Design review of the part built by this model. Coordinates are the model's own, in mm. Face numbers are marked on the shaded views. A direction names the side the tool comes from. Give positions to 0.01 mm unless a question says otherwise; leave off trailing zeros. Loops run counter-clockwise (first coordinate to the right, second up) from the corner with the lowest first, then second, coordinate; pieces in that order, holes last. Notation, with made-up numbers: (-25.75, 3) - (27.25, 3) arc R27 cw to (27.25, 37) - close; hole circle Ø4 at (-21.75, 86.5). An arc over 180 degrees is marked (long way). One line per item, written item: value. Start each with the question number.
```python
from build123d import *

# Parameters (mm, degrees)
SKETCH1_W           = 28.5
SKETCH1_H           = 41.5
SKETCH1_R           = 1.75
BOSS_EXTRUDE1_DEPTH = 1.6
SKETCH2_W           = 2.3
SKETCH2_H           = 9.2
SKETCH2_W_2         = 16
SKETCH2_H_2         = 2.5
BOSS_EXTRUDE2_DEPTH = 9
SKETCH3_W           = 1.5
SKETCH3_H           = 1.5
CUT_EXTRUDE1_DEPTH  = 1
SKETCH4_W           = 6.5
SKETCH4_H           = 6.5
BOSS_EXTRUDE3_DEPTH = 1.1
FILLET1_R           = 0.5
SKETCH5_W           = 7.53
SKETCH5_H           = 5.6
BOSS_EXTRUDE4_DEPTH = 5.3
SKETCH6_W           = 4.23
SKETCH6_H           = 3
CUT_EXTRUDE2_DEPTH  = 4.5


with BuildPart() as part:
    # Sketch1 → Boss-Extrude1 (new body)
    with BuildSketch(Plane(origin=(0, 0, 0), x_dir=(1, 0, 0), z_dir=(0, 1, 0))):
        Rectangle(SKETCH1_W, SKETCH1_H)
        with Locations((11.375, 17.5)):
            Circle(SKETCH1_R, mode=Mode.SUBTRACT)
        with Locations((-11.375, 17.5)):
            Circle(SKETCH1_R, mode=Mode.SUBTRACT)
        with Locations((-11.375, -17.5)):
            Circle(SKETCH1_R, mode=Mode.SUBTRACT)
        with Locations((11.375, -17.5)):
            Circle(SKETCH1_R, mode=Mode.SUBTRACT)
    extrude(amount=BOSS_EXTRUDE1_DEPTH)

    # Sketch2 → Boss-Extrude2 (add)
    with BuildSketch(Plane(origin=(0, 1.6, 0), x_dir=(1, 0, 0), z_dir=(0, 1, 0))):
        with Locations((12.9, 7.15)):
            Rectangle(SKETCH2_W, SKETCH2_H)
        with Locations((9.85, 7.15)):
            Rectangle(SKETCH2_W, SKETCH2_H)
        with Locations((-0.125, 19.4)):
            Rectangle(SKETCH2_W_2, SKETCH2_H_2)
    extrude(amount=BOSS_EXTRUDE2_DEPTH)

    # Sketch3 → Cut-Extrude1 (cut)
    with BuildSketch(Plane(origin=(0, 10.6, 0), x_dir=(1, 0, 0), z_dir=(0, 1, 0))):
        with Locations((12.9, 7.15)):
            Rectangle(SKETCH3_W, SKETCH3_H)
        with Locations((12.9, 9.9)):
            Rectangle(SKETCH3_W, SKETCH3_H)
        with Locations((12.9, 4.9)):
            Rectangle(SKETCH3_W, SKETCH3_H)
        with Locations((9.85, 4.9)):
            Rectangle(SKETCH3_W, SKETCH3_H)
        with Locations((9.85, 7.15)):
            Rectangle(SKETCH3_W, SKETCH3_H)
        with Locations((9.85, 9.9)):
            Rectangle(SKETCH3_W, SKETCH3_H)
        with Locations((6.425, 19.4)):
            Rectangle(SKETCH3_W, SKETCH3_H)
        with Locations((3.885, 19.4)):
            Rectangle(SKETCH3_W, SKETCH3_H)
        with Locations((1.345, 19.4)):
            Rectangle(SKETCH3_W, SKETCH3_H)
        with Locations((-1.195, 19.4)):
            Rectangle(SKETCH3_W, SKETCH3_H)
        with Locations((-3.735, 19.4)):
            Rectangle(SKETCH3_W, SKETCH3_H)
        with Locations((-6.275, 19.4)):
            Rectangle(SKETCH3_W, SKETCH3_H)
    extrude(amount=-CUT_EXTRUDE1_DEPTH, mode=Mode.SUBTRACT)

    # Sketch4 → Boss-Extrude3 (add)
    with BuildSketch(Plane(origin=(0, 1.6, 0), x_dir=(1, 0, 0), z_dir=(0, 1, 0))):
        with Locations((1.45, 7.15)):
            Rectangle(SKETCH4_W, SKETCH4_H)
    extrude(amount=BOSS_EXTRUDE3_DEPTH)

    # Fillet1
    fillet1_edges = [part.edges().sort_by_distance(p)[0] for p in [
        (4.7, 2.7, -7.15),
        (1.45, 2.7, -10.4),
        (-1.8, 2.7, -7.15),
        (1.45, 2.7, -3.9),
    ]]
    fillet(fillet1_edges, radius=FILLET1_R)

    # Sketch5 → Boss-Extrude4 (add)
    with BuildSketch(Plane(origin=(0, 1.6, 0), x_dir=(1, 0, 0), z_dir=(0, 1, 0))):
        with Locations((-4.86, -17.85)):
            Rectangle(SKETCH5_W, SKETCH5_H)
    extrude(amount=BOSS_EXTRUDE4_DEPTH)

    # Sketch6 → Cut-Extrude2 (cut)
    with BuildSketch(Plane.XY.offset(20.65)):
        with Locations((-4.86, 4.25)):
            Rectangle(SKETCH6_W, SKETCH6_H)
    extrude(amount=-CUT_EXTRUDE2_DEPTH, mode=Mode.SUBTRACT)


solid = part.part
```
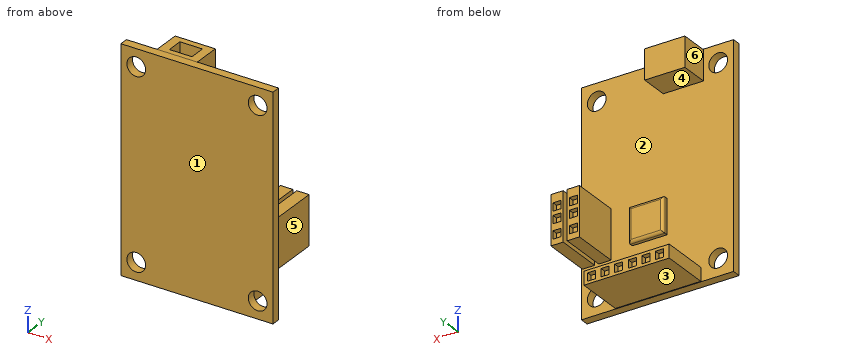
(1) Machinability: for the marked faces 4, 5 and 6, which of the approach directions +Z, -Z, +X, -X, +Y, -Y give a long, thin tool a straight path to every point of the face, cutting with its end or side? Answer none if there is none.
(2) Take a section at B-B on y = 7.5. State the section outline as (x, z) points (3 decimals), and give its area (3 significant figures).
(3) Draft analysis for pull direction Z (two halves, no side actions). For the marked faces 1, 2 and 3, state which applies: pulls with the +Z half, pulls with the -Z half, needs draft (parallel to the pull), parting line crosses it, or undercut.
(4) Take a section at D-D on y = 5. State the section outline as (x, z) points (3 decimals).
(5) To check wall thickness, follow L1, parallel to X at y = 0.3, z = 17.5 (3 decimals); L2, parallel to Z at x = -5.75, y = 4.75; L3, parallel to Z at x = -7, y = 6.75. State the ranges of each line that lie inside material, in increasing order. Write a range as from..to.
(6) For pin 1 Ø0.8 at (y, z) = (10, -19.5) entering from +X (3 decimals); pin 2 Ø0.5 at (x, y) = (13, 10) entering from -Z; pin 3 Ø3 at (x, z) = (-3.5, 7.5) entering from +Y, all flat-tipped, find the tip position at first contact; note any pin that passes through.
(7) Take a section at C-C on x = -5. State the section outline as (y, z) points.
(8) Take a section at A-A on z = 17.5. State the section outline as (x, y) points (3 decimals).
Here are the results:
1. face 4: +X, -X, +Y
1. face 5: +Z, -Z, +X, +Y
1. face 6: +Z, -Z, -X, +Y
2. outline: (-8.125, -20.65) - (7.875, -20.65) - (7.875, -18.15) - (-8.125, -18.15) - close; (8.7, -11.75) - (11, -11.75) - (11, -2.55) - (8.7, -2.55) - close; (11.75, -11.75) - (14.05, -11.75) - (14.05, -2.55) - (11.75, -2.55) - close
2. area: 82.3 mm²
3. face 1: needs draft
3. face 2: undercut
3. face 3: pulls with the -Z half
4. outline: (-8.625, 15.05) - (-1.095, 15.05) - (-1.095, 20.65) - (-2.745, 20.65) - (-2.745, 16.15) - (-6.975, 16.15) - (-6.975, 20.65) - (-8.625, 20.65) - close; (-8.125, -20.65) - (7.875, -20.65) - (7.875, -18.15) - (-8.125, -18.15) - close; (8.7, -11.75) - (11, -11.75) - (11, -2.55) - (8.7, -2.55) - close; (11.75, -11.75) - (14.05, -11.75) - (14.05, -2.55) - (11.75, -2.55) - close
5. L1: -14.25..-13.125, -9.625..9.625, 13.125..14.25
5. L2: -20.65..-18.15, 15.05..16.15
5. L3: -20.65..-18.15, 15.05..20.65
6. pin 1: x = 7.875
6. pin 2: z = -11.75
6. pin 3: y = 1.6
7. outline: (0, -20.75) - (1.6, -20.75) - (1.6, -20.65) - (10.6, -20.65) - (10.6, -18.15) - (1.6, -18.15) - (1.6, 15.05) - (6.9, 15.05) - (6.9, 20.65) - (5.75, 20.65) - (5.75, 16.15) - (2.75, 16.15) - (2.75, 20.65) - (1.6, 20.65) - (1.6, 20.75) - (0, 20.75) - close
8. outline: (-14.25, 0) - (-13.125, 0) - (-13.125, 1.6) - (-14.25, 1.6) - close; (-9.625, 0) - (9.625, 0) - (9.625, 1.6) - (-1.095, 1.6) - (-1.095, 6.9) - (-8.625, 6.9) - (-8.625, 1.6) - (-9.625, 1.6) - close; (13.125, 0) - (14.25, 0) - (14.25, 1.6) - (13.125, 1.6) - close; hole (-6.975, 2.75) - (-2.745, 2.75) - (-2.745, 5.75) - (-6.975, 5.75) - close
